Geometry: final body of the model. Coordinates: model frame, mm. A direction names the side the tool comes from. Coordinates: 2 decimals unless noted, no trailing zeros. Write each loop counter-clockwise with the first axis right and the second up, starting at its lowest first coordinate (ties: lowest second). Pieces come first, ordered by that corner, then holes. Notation, with made-up numbers: (63, 43.5) -> (68, 43.5) arc R10 cw to (68, 53.5) -> close; hole circle Ø7 at (5, 36.25). An arc over 180 degrees is marked (long way). One line per item, written item: value. Start each with the question number.
from build123d import *

# Parameters (mm, degrees)
SKETCH011_W          = 220
SKETCH011_H          = 47.5
SKETCH011_R          = 2.5
PAD006_DEPTH         = 10
SKETCH012_W          = 32
SKETCH012_H          = 47.5
SKETCH012_R          = 3
PAD007_DEPTH         = 7
PAD009_DEPTH         = 44
PAD009_DEPTH_BACK    = 3.5
PAD008_DEPTH         = 3.5
SKETCH015_R          = 2.5
HOLE002_DEPTH        = 15
HOLE002_TIPS_R       = 2.5
SKETCH016_R          = 4.5
POCKET002_DEPTH      = 5
POCKET002_DEPTH_BACK = 100
POCKET003_DEPTH      = 1.5
POCKET003_DEPTH_BACK = 100


with BuildPart() as part:
    # Sketch011 → Pad006 (new body)
    with BuildSketch(Plane.YZ):
        with Locations((110, 20.25)):
            Rectangle(SKETCH011_W, SKETCH011_H)
        with Locations((49.25, 22)):
            Circle(SKETCH011_R, mode=Mode.SUBTRACT)
        with Locations((81.25, 22)):
            Circle(SKETCH011_R, mode=Mode.SUBTRACT)
        with Locations((92.25, 22)):
            Circle(SKETCH011_R, mode=Mode.SUBTRACT)
        with Locations((109.25, 22)):
            Circle(SKETCH011_R, mode=Mode.SUBTRACT)
        with Locations((157.25, 34.5)):
            Circle(SKETCH011_R, mode=Mode.SUBTRACT)
        with Locations((157.25, 9.5)):
            Circle(SKETCH011_R, mode=Mode.SUBTRACT)
        with Locations((182.25, 22)):
            Circle(SKETCH011_R, mode=Mode.SUBTRACT)
    extrude(amount=PAD006_DEPTH)

    # Sketch012 (on Face2 of Pad006) → Pad007 (join)
    with BuildSketch(Plane.XZ):
        with Locations((-6, 20.25)):
            Rectangle(SKETCH012_W, SKETCH012_H)
        with Locations((-8.5, 37)):
            Circle(SKETCH012_R, mode=Mode.SUBTRACT)
        with Locations((-8.5, 22)):
            Circle(SKETCH012_R, mode=Mode.SUBTRACT)
        with Locations((-8.5, 7)):
            Circle(SKETCH012_R, mode=Mode.SUBTRACT)
    extrude(amount=PAD007_DEPTH)

    # Sketch014 → Pad009 (join, two sides)
    with BuildSketch(Plane.XY) as pad009_sk:
        Polygon((0, 2.75), (-22, 2.75), (0, 46.75), align=None)
    extrude(amount=PAD009_DEPTH)
    extrude(pad009_sk.sketch, amount=-PAD009_DEPTH_BACK)

    # Sketch013 → Pad008 (join)
    with BuildSketch(Plane.XY):
        Polygon((10, -7), (10, 153), (46, 153), align=None)
        with BuildLine():
            ThreePointArc((26.75, 142.579156), (24, 141.75), (26.75, 140.920844))
            ThreePointArc((26.75, 140.920844), (29.5, 141.75), (26.75, 142.579156))
        make_face(mode=Mode.SUBTRACT)
    extrude(amount=-PAD008_DEPTH)

    # Sketch015 (on Face21 of Pad008) → Hole002 (cut)
    with BuildSketch(Plane.XZ.offset(-2.75)):
        with Locations((-8.5, 37)):
            Circle(SKETCH015_R)
        with Locations((-8.5, 22)):
            Circle(SKETCH015_R)
        with Locations((-8.5, 7)):
            Circle(SKETCH015_R)
    extrude(amount=-HOLE002_DEPTH, mode=Mode.SUBTRACT)

    # Hole002 tips → Hole002 tip 1 section 0
    with BuildSketch(Plane.XZ.offset(-17.75), mode=Mode.PRIVATE) as hole002_tip_1_s0:
        with Locations((-8.5, 37)):
            Circle(HOLE002_TIPS_R)
    loft([hole002_tip_1_s0.sketch, Vertex(-8.5, 19.252152, 37)], mode=Mode.SUBTRACT)

    # Hole002 tips → Hole002 tip 2 section 0
    with BuildSketch(Plane.XZ.offset(-17.75), mode=Mode.PRIVATE) as hole002_tip_2_s0:
        with Locations((-8.5, 22)):
            Circle(HOLE002_TIPS_R)
    loft([hole002_tip_2_s0.sketch, Vertex(-8.5, 19.252152, 22)], mode=Mode.SUBTRACT)

    # Hole002 tips → Hole002 tip 3 section 0
    with BuildSketch(Plane.XZ.offset(-17.75), mode=Mode.PRIVATE) as hole002_tip_3_s0:
        with Locations((-8.5, 7)):
            Circle(HOLE002_TIPS_R)
    loft([hole002_tip_3_s0.sketch, Vertex(-8.5, 19.252152, 7)], mode=Mode.SUBTRACT)

    # Sketch016 (on Face4 of Hole002) → Pocket002 (cut, two sides)
    with BuildSketch(Plane(origin=(0, 0, 0), x_dir=(0, -1, 0), z_dir=(-1, 0, 0))) as pocket002_sk:
        with Locations((-182.25, 22)):
            Circle(SKETCH016_R)
        with Locations((-157.25, 34.5)):
            Circle(SKETCH016_R)
        with Locations((-157.25, 9.5)):
            Circle(SKETCH016_R)
        with Locations((-109.25, 22)):
            Circle(SKETCH016_R)
        with Locations((-92.25, 22)):
            Circle(SKETCH016_R)
        with Locations((-81.25, 22)):
            Circle(SKETCH016_R)
        with Locations((-49.25, 22)):
            Circle(SKETCH016_R)
    extrude(amount=-POCKET002_DEPTH, mode=Mode.SUBTRACT)
    extrude(pocket002_sk.sketch, amount=POCKET002_DEPTH_BACK, mode=Mode.SUBTRACT)

    # Sketch017 (on Face8 of Pocket002) → Pocket003 (cut, two sides)
    with BuildSketch(Plane(origin=(0, 0, -3.5), x_dir=(1, 0, 0), z_dir=(0, 0, -1))) as pocket003_sk:
        with BuildLine():
            ThreePointArc((26.75, -138.480826), (22, -141.75), (26.75, -145.019174))
            ThreePointArc((26.75, -145.019174), (31.5, -141.75), (26.75, -138.480826))
        make_face()
    extrude(amount=-POCKET003_DEPTH, mode=Mode.SUBTRACT)
    extrude(pocket003_sk.sketch, amount=POCKET003_DEPTH_BACK, mode=Mode.SUBTRACT)


solid = part.part
Q1. Cut plane B-B on x = 2.5. Output: boundary loops of the cut face in (y, z), and give its area (3 significant figures).
Q2. Line query: L1, parallel to Z at x = -8.5, y = 13.25; L2, parallel to Z at x = 7, y = 157.25; L3, parallel to Y at x = 8, z = 22. Output: solid intervals per line, ascending. Write a range as from..to.
Q3. Cut plane D-D on y = 35.5. Output: boundary loops of the cut face in (x, z) (1 decimal).
Q4. Access query for faces 4 (the cylindrical face through (-9.04, 10.14, 34.56)), 5 (the flat face through (-22, -3, 20)), 6 (the flat face through (5, 107, 20)), 7 (the flat face through (20, 110, 0)), 8 (the cylindrical face through (7.46, 159.56, 8.54)). Directions: +Z, -Z, +X, -X, +Y, -Y. A direction counts if a zero-diameter tool reaches every point of the face in a straight line with its end or side. Return the directions, or none.
Q5. First-contact query: P1, Ø6, axis at y = 182.25, z = 22, coming from the -X side; P2, Ø6.5, axis at x = -8.5, z = 22, coming from the -Y side; P3, Ø1.5, axis at y = 64.5, z = 8.5, coming from the +X side; P4, Ø4, axis at y = 187.5, z = 31, coming from the -X side. Flat tips, straight axial feed; report the tip coordinate or a pass-through.
Q6. Cut plane C-C on y = 109.25. Output: boundary loops of the cut face in (x, z).
Q7. Draft query along X for faces 1 (the cylindrical face through (2.465, 113.746, 22.198)), 2 (the flat face through (10, 108, 25)), 3 (the cylindrical face through (31.5, 141.8, -2.8)). Return one class per face: pulls with the +X half, pulls with the -X half, needs draft (parallel to the pull), parting line crosses it, or undercut.
Q8. Cut plane A-A on y = 157.25. Output: boundary loops of the cut face in (x, z), and give its area (3 significant figures).
Solution:
1. outline: (-7, -3.5) -> (220, -3.5) -> (220, 44) -> (-7, 44) -> close; hole circle Ø9 at (49.25, 22); hole circle Ø9 at (81.25, 22); hole circle Ø9 at (92.25, 22); hole circle Ø9 at (109.25, 22); hole circle Ø9 at (157.25, 9.5); hole circle Ø9 at (157.25, 34.5); hole circle Ø9 at (182.25, 22)
1. area: 10,300 mm²
2. L1: -3.5..4.5, 9.5..19.5, 24.5..34.5, 39.5..44
2. L2: -3.5..7, 12..32, 37..44
2. L3: -7..46.75, 51.75..78.75, 83.75..89.75, 94.75..106.75, 111.75..179.75, 184.75..220
3. outline: (-5.6, -3.5) -> (19.6, -3.5) -> (19.6, 0) -> (10, 0) -> (10, 44) -> (-5.6, 44) -> close
4. face 4: -Y
4. face 5: +Z, -Z, -X, +Y, -Y
4. face 6: -X
4. face 7: +Z, +X, +Y, -Y
4. face 8: +X, -X
5. P1: x = 5
5. P2: y = -7
5. P3: x = 10
5. P4: x = 0
6. outline: (0, -3.5) -> (36.16, -3.5) -> (36.16, 0) -> (10, 0) -> (10, 19.5) -> (5, 19.5) -> (5, 17.5) -> (0, 17.5) -> close; (0, 26.5) -> (5, 26.5) -> (5, 24.5) -> (10, 24.5) -> (10, 44) -> (0, 44) -> close
7. face 1: needs draft
7. face 2: pulls with the +X half
7. face 3: undercut
8. outline: (0, -3.5) -> (10, -3.5) -> (10, 7) -> (5, 7) -> (5, 5) -> (0, 5) -> close; (0, 14) -> (5, 14) -> (5, 12) -> (10, 12) -> (10, 32) -> (5, 32) -> (5, 30) -> (0, 30) -> close; (0, 39) -> (5, 39) -> (5, 37) -> (10, 37) -> (10, 44) -> (0, 44) -> close
8. area: 335 mm²
